Work out the finished part from the listing and answer in its coordinate system (mm). A direction names the side the tool comes from. Give positions to 0.01 mm unless a question says otherwise; leave off trailing zeros. Order: outer loops, then holes, each group sorted by start corner. A loop starts at its lowest first (then second) coordinate and runs counter-clockwise, first axis right, second up. Notation, with made-up numbers: (15, 38.5) -> (42, 38.5) arc R19 cw to (42, 53.5) -> close; hole circle Ø6 at (67, 69). An arc over 180 degrees is marked (long way). Answer as CSV lines item,"result". Start each with the question number.
1. A cutting plane is placed at A-A (x = 0). Give the vertices of the cut face in (y, z).
2. Find the intervals of material crossed by L1, parallel to Z at x = 0.4, y = -1.3; L2, parallel to Y at x = -0.9, z = 1.25; L3, parallel to Z at x = 0.1, y = -2.7, in increasing order.
3. For a pull along Y with two mould halves and no side action, classify faces 3 (the cylindrical face through (1.5, 0.07, -3.04)), 4 (the flat face through (0, 0, -6)), 5 (the flat face through (1.305, 0.74, 1.155)) as released by +Y, released by -Y, zero draft, split by the parting line, or undercut.
4. A cutting plane is placed at B-B (z = -3.5). Give the vertices of the cut face in (x, y).
5. Flat-ended cylindrical pins translate along their axes: pin 1 (1.5 mm diameter, centred on x = 0.5, z = -2.5, fed in from -Y); pin 2 (2 mm diameter, centred on x = 2, y = -2, fed in from -Z); pin 3 (2 mm diameter, centred on x = 0.5, z = -3.5, fed in from +Y); pin 4 (2.5 mm diameter, centred on x = 0, y = -0.5, fed in from +Z). Find the tip coordinate at first contact, or state that the pin passes through.
6. For faces 1 (the flat face through (1.3, -1.3, 1.5)), 2 (the flat face through (0, 0, 0.8)), determine the directions among +Z, -Z, +X, -X, +Y, -Y from which every point of the face is accessible in a straight line to the end or side of a thin tool.
from build123d import *

# Parameters (mm, degrees)
F3_DEPTH = 0.7


with BuildPart() as f1:
    # F0 (on Front) → F1 (revolve)
    with BuildSketch(Plane.XZ):
        Polygon((-1.5, 0), (-1.5, -6), (0, -6), (0, 1.5), (-3, 1.5), align=None)
    revolve(axis=Axis((0, 0, -4.202494), (0, 0, -1)))

    # F2 (on face) → F3 (cut)
    with BuildSketch(Plane.XY.offset(1.5)):
        Polygon((-0.866025, -1.5), (0.866025, -1.5), (1.732051, 0), (0.866025, 1.5), (-0.866025, 1.5), (-1.732051, 0), align=None)
    extrude(amount=-F3_DEPTH, mode=Mode.SUBTRACT)


solid = f1.part
Answer sheet:
1,outline,"(-3, 1.5) -> (-1.5, 0) -> (-1.5, -6) -> (1.5, -6) -> (1.5, 0) -> (3, 1.5) -> (1.5, 1.5) -> (1.5, 0.8) -> (-1.5, 0.8) -> (-1.5, 1.5) -> close"
2,L1,"z = -6 to 0.8"
2,L2,"y = -2.6 to -1.44, 1.44 to 2.6"
2,L3,"z = 1.2 to 1.5"
3,face 3,"split by the parting line"
3,face 4,"zero draft"
3,face 5,"undercut"
4,outline,"circle Ø3 at (0, 0)"
5,pin 1,"stops at y = -1.5"
5,pin 2,"stops at z = 0.33"
5,pin 3,"stops at y = 1.5"
5,pin 4,"stops at z = 1.5"
6,face 1,"+Z, +X, -X, +Y, -Y"
6,face 2,"+Z"
